Build history of the part. All positions in model axes, mm. Give positions to 0.01 mm unless a question says otherwise; leave off trailing zeros. Loops run counter-clockwise (first coordinate to the right, second up) from the corner with the lowest first, then second, coordinate; pieces in that order, holes last. Notation, with made-up numbers: (-21, 74.25) -> (31, 74.25) arc R21 cw to (31, 97.25) -> close; hole circle Ø3 at (75.5, 56.25). An arc over 180 degrees is marked (long way). Answer as a JSON object with one key per item and string values. Group by question number.
Q1. Band-saw the part on C-C, the plane x = -8. Write the cut outline in (y, z).
Q2. Wall check: probe 1 along Y at (x, z) = (-17, 0.2); probe 2 along Y at (x, z) = (12, 2.75); probe 3 along X at (y, z) = (36, 1.65). Give the ranges that are in metal, low to high. Write a range as from..to.
Q3. Band-saw the part on D-D, the plane y = 48. Write the cut outline in (x, z), plus the area to 3 significant figures.
Q4. Drop flat-ended pins along their axis: pin 1 (8.5 mm diameter, centred on x = 8, y = 79, fed in from +Z); pin 2 (1.5 mm diameter, centred on x = 22, z = 2.5, fed in from -Y). Give the stop position or say it passes through.
Q5. Band-saw the part on B-B, the plane x = -23. Write the cut outline in (y, z).
Q6. Band-saw the part on A-A, the plane y = 5. Write the cut outline in (x, z), plus the area to 3 significant figures.
from build123d import *

# Parameters (mm, degrees)
SKETCH1_R           = 2.915712225
SKETCH1_R_2         = 2.67310125
SKETCH1_R_3         = 3
SKETCH1_R_4         = 10
BOSS_EXTRUDE2_DEPTH = 3
FILLET1_R           = 4


with BuildPart() as part:
    # Sketch1 → Boss-Extrude2 (new body)
    with BuildSketch(Plane.XY):
        Polygon((17.4253449, 0), (-17.4253449, 0), (-35, 26.741942676), (-35, 66.741942676), (-18, 85), (18, 85), (35, 66.741942676), (35, 26.741942676), align=None)
        with Locations((-23, 53)):
            Circle(SKETCH1_R, mode=Mode.SUBTRACT)
        with Locations((-8, 79)):
            Circle(SKETCH1_R_2, mode=Mode.SUBTRACT)
        with Locations((-8, 7)):
            Circle(SKETCH1_R_3, mode=Mode.SUBTRACT)
        with Locations(Location((8, 7, 0), (0, 0, 180))):
            Circle(SKETCH1_R_3, mode=Mode.SUBTRACT)
        with Locations(Location((23, 53, 0), (0, 0, 180))):
            Circle(SKETCH1_R, mode=Mode.SUBTRACT)
        with Locations(Location((8, 79, 0), (0, 0, 180))):
            Circle(SKETCH1_R_2, mode=Mode.SUBTRACT)
        with Locations((8.931523687, 26.741942676)):
            Circle(SKETCH1_R_4, mode=Mode.SUBTRACT)
        with BuildLine():
            Line((-14.43882876, 55.489231101), (14.43882876, 55.489231101))
            ThreePointArc((14.43882876, 55.489231101), (15.957952298, 58.468042486), (18.467610338, 60.677718959))
            ThreePointArc((18.467610338, 60.677718959), (0, 73), (-18.467610338, 60.677718959))
            ThreePointArc((-18.467610338, 60.677718959), (-15.957952298, 58.468042486), (-14.43882876, 55.489231101))
        make_face(mode=Mode.SUBTRACT)
        with BuildLine():
            Line((-14.43882876, 50.510768899), (14.43882876, 50.510768899))
            ThreePointArc((14.43882876, 50.510768899), (15.957952298, 47.531957514), (18.467610338, 45.322281041))
            ThreePointArc((18.467610338, 45.322281041), (19.38241537, 41.987278709), (16.047413038, 41.072473676))
            ThreePointArc((16.047413038, 41.072473676), (0.501050083, 40.340733608), (-7.068476313, 26.741942676))
            ThreePointArc((-7.068476313, 26.741942676), (-12.768043325, 21.042375664), (-18.467610338, 26.741942676))
            Line((-18.467610338, 26.741942676), (-18.467610338, 45.322281041))
            ThreePointArc((-18.467610338, 45.322281041), (-15.957952298, 47.531957514), (-14.43882876, 50.510768899))
        make_face(mode=Mode.SUBTRACT)
    extrude(amount=BOSS_EXTRUDE2_DEPTH)

    # Fillet1
    fillet1_edges = [part.edges().sort_by_distance(p)[0] for p in [
        (-35, 26.741942676, 1.5),
        (-35, 66.741942676, 1.5),
        (-18, 85, 1.5),
        (18, 85, 1.5),
        (35, 66.741942676, 1.5),
        (35, 26.741942676, 1.5),
        (17.4253449, 0, 1.5),
        (-17.4253449, 0, 1.5),
    ]]
    fillet(fillet1_edges, radius=FILLET1_R)


solid = part.part
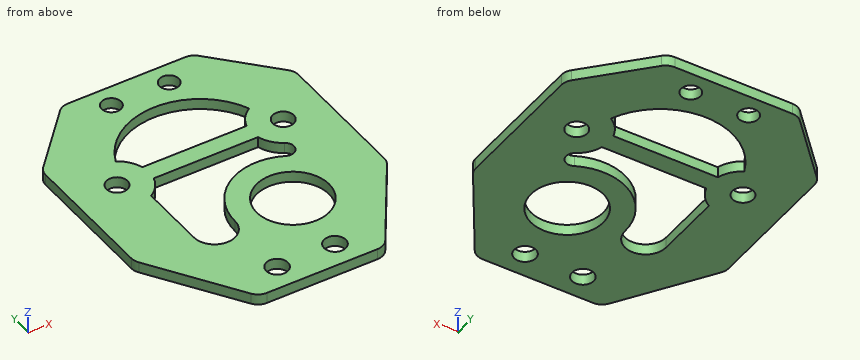
Worked answers:
{
 "1": {"outline": "(0, 0) -> (4, 0) -> (4, 3) -> (0, 3) -> close; (10, 0) -> (23.62, 0) -> (23.62, 3) -> (10, 3) -> close; (50.51, 0) -> (55.49, 0) -> (55.49, 3) -> (50.51, 3) -> close; (71.33, 0) -> (76.33, 0) -> (76.33, 3) -> (71.33, 3) -> close; (81.67, 0) -> (85, 0) -> (85, 3) -> (81.67, 3) -> close"},
 "2": {"probe 1": "0.39..22.92, 46.41..59.59, 63.54..84.93", "probe 2": "0..17.22, 36.26..42.44, 50.51..55.49, 69..85", "probe 3": "-35..-18.47, -4.12..5.15, 12.71..35"},
 "3": {"outline": "(-35, 0) -> (-15.62, 0) -> (-15.62, 3) -> (-35, 3) -> close; (15.62, 0) -> (35, 0) -> (35, 3) -> (15.62, 3) -> close", "area": "116 mm2"},
 "4": {"pin 1": "z = 3", "pin 2": "y = 5.82"},
 "5": {"outline": "(8.48, 0) -> (50.08, 0) -> (50.08, 3) -> (8.48, 3) -> close; (55.92, 0) -> (79.63, 0) -> (79.63, 3) -> (55.92, 3) -> close"},
 "6": {"outline": "(-20.71, 0) -> (-10.24, 0) -> (-10.24, 3) -> (-20.71, 3) -> close; (-5.76, 0) -> (5.76, 0) -> (5.76, 3) -> (-5.76, 3) -> close; (10.24, 0) -> (20.71, 0) -> (20.71, 3) -> (10.24, 3) -> close", "area": "97.4 mm2"}
}
